```python
from build123d import *

# Parameters (mm, degrees)
SKETCH1_W           = 3.6
SKETCH1_H           = 2.8
BOSS_EXTRUDE1_DEPTH = 0.4
SKETCH2_W           = 0.4
SKETCH2_H           = 1.8
BOSS_EXTRUDE2_DEPTH = 0.7
SKETCH3_W           = 0.4
SKETCH3_H           = 1.8
BOSS_EXTRUDE3_DEPTH = 0.7
SKETCH4_W           = 3.1
SKETCH4_H           = 2.8
BOSS_EXTRUDE4_DEPTH = 0.5
SKETCH5_W           = 5.5
SKETCH5_H           = 3.1
BOSS_EXTRUDE5_DEPTH = 1.7
SKETCH6_W           = 3.1
SKETCH6_H           = 4.5
BOSS_EXTRUDE6_DEPTH = 0.5
SKETCH7_W           = 6
SKETCH7_H           = 4.5
BOSS_EXTRUDE7_DEPTH = 0.4
SKETCH8_W           = 5
SKETCH8_H           = 2.7
CUT_EXTRUDE1_DEPTH  = 0.6
BOSS_EXTRUDE8_DEPTH = 5
CUT_EXTRUDE2_REACH  = 8
SKETCH10_W          = 0.8
SKETCH10_H          = 1.8
SKETCH11_W          = 0.8
SKETCH11_H          = 1.8
CUT_EXTRUDE3_DEPTH  = 7
SKETCH12_W          = 0.25
SKETCH12_H          = 2.7
SKETCH13_W          = 0.25
SKETCH13_H          = 2.7
SKETCH14_W          = 0.25
SKETCH14_H          = 2.7
SKETCH15_W          = 0.25
SKETCH15_H          = 2.4
SKETCH16_W          = 0.25
SKETCH16_H          = 2.4
SKETCH17_W          = 0.25
SKETCH17_H          = 2.4


with BuildPart() as part:
    # Sketch1 → Boss-Extrude1 (new body)
    with BuildSketch(Plane.XY):
        with Locations((0, 3.1)):
            Rectangle(SKETCH1_W, SKETCH1_H)
    extrude(amount=-BOSS_EXTRUDE1_DEPTH)

    # Sketch2 → Boss-Extrude2 (add)
    with BuildSketch(Plane.ZY.offset(1.8)):
        with Locations((-0.2, 3.6)):
            Rectangle(SKETCH2_W, SKETCH2_H)
    extrude(amount=BOSS_EXTRUDE2_DEPTH)

    # Sketch3 → Boss-Extrude3 (add)
    with BuildSketch(Plane(origin=(1.8, 0, 0), x_dir=(0, 0, -1), z_dir=(1, 0, 0))):
        with Locations((0.2, 3.6)):
            Rectangle(SKETCH3_W, SKETCH3_H)
    extrude(amount=BOSS_EXTRUDE3_DEPTH)

    # Sketch4 → Boss-Extrude4 (add)
    with BuildSketch(Plane(origin=(2.5, 0, 0), x_dir=(0, 0, -1), z_dir=(1, 0, 0))):
        with Locations((1.55, 3.1)):
            Rectangle(SKETCH4_W, SKETCH4_H)
    extrude(amount=BOSS_EXTRUDE4_DEPTH)

    # Sketch5 → Boss-Extrude5 (add)
    with BuildSketch(Plane.XZ.offset(-1.7)):
        with Locations((0.25, -1.55)):
            Rectangle(SKETCH5_W, SKETCH5_H)
    extrude(amount=BOSS_EXTRUDE5_DEPTH)

    # Sketch6 → Boss-Extrude6 (add)
    with BuildSketch(Plane.ZY.offset(2.5)):
        with Locations((-1.55, 2.25)):
            Rectangle(SKETCH6_W, SKETCH6_H)
    extrude(amount=BOSS_EXTRUDE6_DEPTH)

    # Sketch7 → Boss-Extrude7 (add)
    with BuildSketch(Plane(origin=(0, 0, -3.1), x_dir=(-1, 0, 0), z_dir=(0, 0, -1))):
        with Locations((0, 2.25)):
            Rectangle(SKETCH7_W, SKETCH7_H)
    extrude(amount=BOSS_EXTRUDE7_DEPTH)

    # Sketch8 → Cut-Extrude1 (cut)
    with BuildSketch(Plane(origin=(0, 1.7, 0), x_dir=(-1, 0, 0), z_dir=(0, 1, 0))):
        with Locations((0, -1.75)):
            Rectangle(SKETCH8_W, SKETCH8_H)
    extrude(amount=-CUT_EXTRUDE1_DEPTH, mode=Mode.SUBTRACT)

    # Sketch9 → Boss-Extrude8 (add)
    with BuildSketch(Plane.ZY.offset(-2.5)):
        Polygon((-0.4, 1.4), (-0.4, 1.1), (-2.05, 1.1), (-1.75, 1.4), align=None)
    extrude(amount=BOSS_EXTRUDE8_DEPTH)

    # Sketch10 → Cut-Extrude2 (cut, up to next)
    with BuildSketch(Plane(origin=(3, 0, 0), x_dir=(0, 0, -1), z_dir=(1, 0, 0)), mode=Mode.PRIVATE) as cut_extrude2_sk1:
        with Locations((1.35, 3.6)):
            Rectangle(SKETCH10_W, SKETCH10_H)
    cut_extrude2_tool1 = extrude(cut_extrude2_sk1.sketch, amount=-CUT_EXTRUDE2_REACH, mode=Mode.PRIVATE) & part.part
    add(cut_extrude2_tool1.solids().sort_by_distance((3, 3.6, -1.35))[0], mode=Mode.SUBTRACT)

    # Sketch11 → Cut-Extrude3 (cut, through all)
    with BuildSketch(Plane.ZY.offset(3)):
        with Locations((-1.35, 3.6)):
            Rectangle(SKETCH11_W, SKETCH11_H)
    extrude(amount=-CUT_EXTRUDE3_DEPTH, mode=Mode.SUBTRACT)

    # Sketch12 → Revolve1 (revolve)
    with BuildSketch(Plane(origin=(0, 0, -1.3), x_dir=(-1, 0, 0), z_dir=(0, 0, -1))):
        with Locations((1.375, -1.35)):
            Rectangle(SKETCH12_W, SKETCH12_H)
    revolve(axis=Axis((-1.5, -2.7, -1.3), (0, 1, 0)))

    # Sketch13 → Revolve2 (revolve)
    with BuildSketch(Plane(origin=(0, 0, -1.3), x_dir=(-1, 0, 0), z_dir=(0, 0, -1))):
        with Locations((-0.125, -1.35)):
            Rectangle(SKETCH13_W, SKETCH13_H)
    revolve(axis=Axis((0, -2.7, -1.3), (0, 1, 0)))

    # Sketch14 → Revolve3 (revolve)
    with BuildSketch(Plane(origin=(0, 0, -1.3), x_dir=(-1, 0, 0), z_dir=(0, 0, -1))):
        with Locations((-1.625, -1.35)):
            Rectangle(SKETCH14_W, SKETCH14_H)
    revolve(axis=Axis((1.5, -2.7, -1.3), (0, 1, 0)))

    # Sketch15 → Revolve4 (revolve)
    with BuildSketch(Plane(origin=(0, 0, -1.3), x_dir=(-1, 0, 0), z_dir=(0, 0, -1))):
        with Locations((-1.625, 2.6)):
            Rectangle(SKETCH15_W, SKETCH15_H)
    revolve(axis=Axis((1.5, 1.4, -1.3), (0, 1, 0)))

    # Sketch16 → Revolve5 (revolve)
    with BuildSketch(Plane(origin=(0, 0, -1.3), x_dir=(-1, 0, 0), z_dir=(0, 0, -1))):
        with Locations((-0.125, 2.6)):
            Rectangle(SKETCH16_W, SKETCH16_H)
    revolve(axis=Axis((0, 1.4, -1.3), (0, 1, 0)))

    # Sketch17 → Revolve6 (revolve)
    with BuildSketch(Plane(origin=(0, 0, -1.3), x_dir=(-1, 0, 0), z_dir=(0, 0, -1))):
        with Locations((1.375, 2.6)):
            Rectangle(SKETCH17_W, SKETCH17_H)
    revolve(axis=Axis((-1.5, 1.4, -1.3), (0, 1, 0)))


solid = part.part
```
Geometry check sheet. Reference: the model listing, model coordinates, mm. A direction names the side the tool comes from. Round coordinates to 2 decimals unless told otherwise and drop trailing zeros. Order: outer loops, then holes, each group sorted by start corner. A loop starts at its lowest first (then second) coordinate and runs counter-clockwise, first axis right, second up. Notation, with made-up numbers: (19, -20.5) -> (24, -20.5) arc R17 ccw to (24, 12.5) -> close; hole circle Ø4 at (-18.75, 37). An arc over 180 degrees is marked (long way). Return JSON: item names as keys, results as strings. Group by question number.
Q1. Material ranges on probe 1 along Z at (x, y) = (0.5, 3.5); probe 2 along X at (y, z) = (1.25, -2.55); probe 3 along Y at (x, z) = (-0.3, -1.1), recorded low to high. Write a range as from..to.
Q2. Gauge pin test, flat end, axial feed: pin 1 (1 mm diameter, centred on x = 1, z = -0.5, fed in from -Y). Record the tip position at first contact, or that the pin passes through.
Q3. Section check D-D, the plane y = -1. Record the boundary of the cut face in (x, z).
Q4. Tool access check on faces 4 (the flat face through (3, 2, -2)), 5 (the flat face through (0, 1.4, -0.9)). Record the directions out of +Z, -Z, +X, -X, +Y, -Y that give a thin tool (end or side, any length) a straight path to the whole face; none if there is none.
Q5. Section check B-B, the plane x = 0.55. Record the boundary of the cut face in (y, z), plus the area to 3 significant figures.
Q6. Release check for a two-part mould opening along X. For faces 1 (the flat face through (0, 2, -3.5)), 2 (the flat face through (-3, 2, -2)), 3 (the flat face through (2.5, 3, -2)) record: released by +X, released by -X, zero draft, split by the parting line, or undercut.
Q7. Section check C-C, the plane z = -2.15. Record the boundary of the cut face in (x, y).
Q8. Section check A-A, the plane y = 4.25. Record the boundary of the cut face in (x, z), plus the area to 3 significant figures.
Numbers:
{
 "1": {"probe 1": "-3.5..-3.1, -0.4..0", "probe 2": "-3..-2.5, 2.5..3", "probe 3": "0..1.4"},
 "2": {"pin 1": "y = 0"},
 "3": {"outline": "circle Ø0.5 at (-1.5, -1.3); circle Ø0.5 at (0, -1.3); circle Ø0.5 at (1.5, -1.3)"},
 "4": {"face 4": "+Z, -Z, +X, +Y, -Y", "face 5": "+Y"},
 "5": {"outline": "(0, -3.5) -> (4.5, -3.5) -> (4.5, -3.1) -> (1.1, -3.1) -> (1.1, -2.05) -> (1.4, -1.75) -> (1.4, -0.4) -> (4.5, -0.4) -> (4.5, 0) -> (0, 0) -> close", "area": "7.02 mm^2"},
 "6": {"face 1": "zero draft", "face 2": "released by -X", "face 3": "undercut"},
 "7": {"outline": "(-3, 0) -> (3, 0) -> (3, 4.5) -> (2.5, 4.5) -> (2.5, 1.1) -> (-2.5, 1.1) -> (-2.5, 4.5) -> (-3, 4.5) -> close"},
 "8": {"outline": "(-3, -3.5) -> (3, -3.5) -> (3, -1.75) -> (2.5, -1.75) -> (2.5, -3.1) -> (-2.5, -3.1) -> (-2.5, -1.75) -> (-3, -1.75) -> close; (-3, -0.95) -> (-2.5, -0.95) -> (-2.5, -0.4) -> (2.5, -0.4) -> (2.5, -0.95) -> (3, -0.95) -> (3, 0) -> (-3, 0) -> close", "area": "6.70 mm^2"}
}
